from build123d import *

# Parameters (mm, degrees)
SKETCH1_R               = 3.175
BOSS_EXTRUDE1_DEPTH     = 38.1
SKETCH2_R               = 7.237173009
CUT_EXTRUDE1_DEPTH      = 4.7625
CUT_EXTRUDE2_DEPTH      = 39.363670966
CUT_EXTRUDE2_DEPTH_BACK = 39.363670966
SKETCH4_R               = 0.8255
SKETCH5_R               = 3.175
SKETCH5_R_2             = 2.916705682
CUT_EXTRUDE3_DEPTH      = 0.635


with BuildPart() as part:
    # Sketch1 → Boss-Extrude1 (new, symmetric)
    with BuildSketch(Plane(origin=(0, 0, 0), x_dir=(1, 0, 0), z_dir=(0, 1, 0))):
        with Locations(Location((0, 0, 0), (0, 0, 90))):
            Circle(SKETCH1_R)
    extrude(amount=BOSS_EXTRUDE1_DEPTH, both=True)

    # Sketch2 → Cut-Extrude1 (cut)
    with BuildSketch(Plane.XZ.offset(38.1)):
        with Locations((0, 0.163997739)):
            Circle(SKETCH2_R)
    extrude(amount=-CUT_EXTRUDE1_DEPTH, mode=Mode.SUBTRACT)

    # Sketch4 → Cut-Extrude2 (cut, two sides: drawn at the far end of the back side and taken through both)
    with BuildSketch(Plane.XY.offset(-CUT_EXTRUDE2_DEPTH_BACK)):
        with Locations((0, 31.489271019)):
            Circle(SKETCH4_R)
        with Locations((0, -31.74365)):
            Circle(SKETCH4_R)
    extrude(amount=CUT_EXTRUDE2_DEPTH + CUT_EXTRUDE2_DEPTH_BACK, mode=Mode.SUBTRACT)

    # Sketch5 → Cut-Extrude3 (cut)
    with BuildSketch(Plane.XZ.offset(7.6073)):
        with Locations(Location((0, 0, 0), (0, 0, 270))):
            Circle(SKETCH5_R)
        Circle(SKETCH5_R_2, mode=Mode.SUBTRACT)
    extrude(amount=CUT_EXTRUDE3_DEPTH, mode=Mode.SUBTRACT)


solid = part.part
Can you work these out from the model? Positions are in its coordinate system, mm. A direction names the side the tool comes from. Give positions to 0.01 mm unless a question says otherwise; leave off trailing zeros. Write each loop counter-clockwise with the first axis right and the second up, starting at its lowest first coordinate (ties: lowest second). Pieces come first, ordered by that corner, then holes. Notation, with made-up numbers: M 82.5,-34.75 L 98.5,-34.75 A16 cw 98.5,-26.75 Z; hole C 12.5,29 d9. An arc over 180 degrees is marked long. Answer in a Markdown table with one row per item. Add a question column.
Item 1: Please list where these lines run through material, in increasing order: L1, parallel to Y at x = 0, z = -1.5; L2, parallel to Y at x = -0.75, z = -1.25; L3, parallel to X at y = 32, z = 2.25.
Item 2: Imagine slicing it at C-C, the plane y = 21.5. Write out the boundary of the cut face in (x, z) (3 decimals), plus the area to 3 significant figures.
Item 3: For pin 1 Ø1.3 at (x, y) = (0, -31.74) entering from -Z, with a flat end and sliding along its axis, tell me the tip position at first contact or that it passes through.
Item 4: Imagine slicing it at D-D, the plane z = -1.5. Write out the boundary of the cut face in (x, y), plus the area to 3 significant figures.
Item 5: Imagine slicing it at B-B, the plane z = 1.75. Write out the boundary of the cut face in (x, y).
Item 6: On a 3-axis mill with a long thin cutter (end or side, diameter ignored), from which of +Z, -Z, +X, -X, +Y, -Y can I reach the whole of each face in a straight line? I mean faces 1 (the cylindrical face through (1.22, -20.61, -2.93)), 2 (the cylindrical face through (-0.632, -7.92, -2.847)). Say none if no direction works.
Item 7: Imagine slicing it at A-A, the plane x = 0. State how many separate pieces and enclosed holes the cut face has, plus the area to 3 significant figures.
Evaluation:
| question | item | result |
|---|---|---|
| 1 | L1 | y = -33.34 to -32.57, -30.92 to 30.66, 32.31 to 38.1 |
| 1 | L2 | y = -33.34 to -32.09, -31.4 to 31.14, 31.83 to 38.1 |
| 1 | L3 | x = -2.24 to -0.65, 0.65 to 2.24 |
| 2 | outline | C 0,0 d6.35 |
| 2 | area | 31.7 mm² |
| 3 | pin 1 | passes through |
| 4 | outline | M -2.8,-33.34 L 2.8,-33.34 L 2.8,-8.24 L 2.5,-8.24 L 2.5,-7.61 L 2.8,-7.61 L 2.8,38.1 L -2.8,38.1 L -2.8,-7.61 L -2.5,-7.61 L -2.5,-8.24 L -2.8,-8.24 Z; hole C 0,-31.74 d1.65; hole C 0,31.49 d1.65 |
| 4 | area | 395 mm² |
| 5 | outline | M -2.65,-33.34 L 2.65,-33.34 L 2.65,-8.24 L 2.33,-8.24 L 2.33,-7.61 L 2.65,-7.61 L 2.65,38.1 L -2.65,38.1 L -2.65,-7.61 L -2.33,-7.61 L -2.33,-8.24 L -2.65,-8.24 Z; hole C 0,-31.74 d1.65; hole C 0,31.49 d1.65 |
| 6 | face 1 | +Y, -Y |
| 6 | face 2 | none |
| 7 | separate pieces | 3 |
| 7 | enclosed holes | 0 |
| 7 | area | 432 mm² |
